Here's how the part is built. I have some questions about the finished solid (model axes, mm). Coordinates: 2 decimals unless noted, no trailing zeros. Write each loop counter-clockwise with the first axis right and the second up, starting at its lowest first coordinate (ties: lowest second). Pieces come first, ordered by that corner, then holes.
(1) Please list where these lines run through material, in increasing order: probe 1 along X at (y, z) = (-0.1, 0); probe 2 along Z at (x, y) = (0, 0.15); probe 3 along X at (y, z) = (0.3, -1.5).
(2) Imagine slicing it at B-B, the plane x = -2.5. List the corners of the cut face in (y, z) for me.
(3) Imagine slicing it at D-D, the plane x = -3.5. List the corners of the cut face in (y, z) for me, plus the area to 3 significant figures.
(4) Imagine slicing it at C-C, the plane x = 0. List the corners of the cut face in (y, z) for me.
(5) Imagine slicing it at A-A, the plane z = 1. List the corners of the cut face in (x, y) for me.
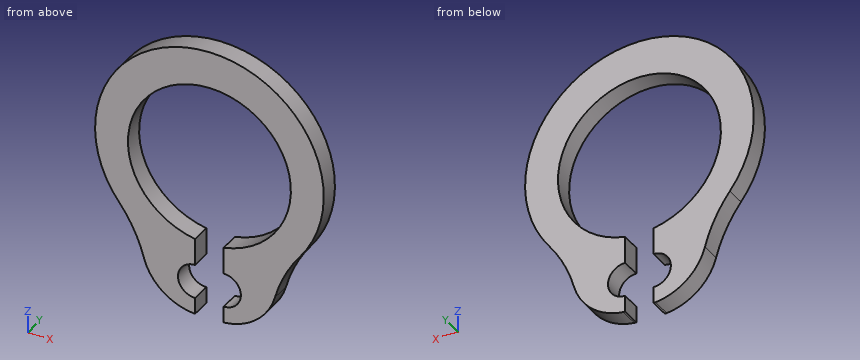
```python
from build123d import *

# Parameters (mm, degrees)
F1_DEPTH    = 0.35
F2_T1_DEPTH = 0.7
F3_R        = 2


# Not quite as in the source:
# - a fillet or chamfer that OpenCascade refuses, or shapes differently, is made with other operations: its cross-section is extruded or revolved along the edge and cut away or added


with BuildPart() as f1:
    # F0 (on Front) → F1 (new body, symmetric)
    with BuildSketch(Plane.XZ):
        with BuildLine():
            ThreePointArc((-0.5, -2.8057975693), (0, 2.85), (0.5, -2.8057975693))
            Line((0.5, -2.8057975693), (0.5, -3.75))
            ThreePointArc((0.5, -3.75), (1.1, -4.35), (0.5, -4.95))
            Line((0.5, -4.95), (0.5, -5.5274315916))
            ThreePointArc((0.5, -5.5274315916), (1.3270959738, -5.3889995617), (2.1238930496, -5.1275314054))
            Line((2.1238930496, -5.1275314054), (1.4775430927, -3.5671045734))
            ThreePointArc((1.4775430927, -3.5671045734), (0, 4.15), (-1.4775430927, -3.5671045734))
            Line((-1.4775430927, -3.5671045734), (-2.1238930496, -5.1275314054))
            ThreePointArc((-2.1238930496, -5.1275314054), (-1.3270959738, -5.3889995617), (-0.5, -5.5274315916))
            Line((-0.5, -5.5274315916), (-0.5, -4.95))
            ThreePointArc((-0.5, -4.95), (-1.1, -4.35), (-0.5, -3.75))
            Line((-0.5, -3.75), (-0.5, -2.8057975693))
        make_face()
    extrude(amount=F1_DEPTH, both=True)

    # F2: fillet of radius 5 on 2 edges, made by hand

    # F2_s2 → F2_t1 (join)
    with BuildSketch(Plane.XZ.offset(-0.35)):
        with BuildLine():
            ThreePointArc((3.163836873, -2.2974754832), (2.4254620947, -3.6322482415), (2.1238930496, -5.1275314054))
            Line((2.1238930496, -5.1275314054), (1.4775430927, -3.5671045734))
            ThreePointArc((1.4775430927, -3.5671045734), (2.4059491896, -3.0455294549), (3.163836873, -2.2974754832))
        make_face()
        with BuildLine():
            ThreePointArc((-2.1238930496, -5.1275314054), (-2.4254620947, -3.6322482415), (-3.163836873, -2.2974754832))
            ThreePointArc((-3.163836873, -2.2974754832), (-2.4059491896, -3.0455294549), (-1.4775430927, -3.5671045734))
            Line((-1.4775430927, -3.5671045734), (-2.1238930496, -5.1275314054))
        make_face()
    extrude(amount=F2_T1_DEPTH)

    # F3
    f3_edges = [f1.edges().sort_by_distance(p)[0] for p in [
        (-2.123893, 0, -5.127531),
        (2.123893, 0, -5.127531),
    ]]
    fillet(f3_edges, radius=F3_R)


solid = f1.part
```
Recorded:
1. probe 1: x = -4 to -2.85, 2.85 to 4
1. probe 2: z = 2.85 to 4.15
1. probe 3: x = -3.64 to -2.42, 2.42 to 3.64
2. outline: (-0.35, -3.44) - (0.35, -3.44) - (0.35, -1.37) - (-0.35, -1.37) - close; (-0.35, 1.37) - (0.35, 1.37) - (0.35, 3.27) - (-0.35, 3.27) - close
3. outline: (-0.35, -1.79) - (0.35, -1.79) - (0.35, 2.09) - (-0.35, 2.09) - close
3. area: 2.71 mm2
4. outline: (-0.35, 2.85) - (0.35, 2.85) - (0.35, 4.15) - (-0.35, 4.15) - close
5. outline: (-3.91, -0.35) - (-2.67, -0.35) - (-2.67, 0.35) - (-3.91, 0.35) - close; (2.67, -0.35) - (3.91, -0.35) - (3.91, 0.35) - (2.67, 0.35) - close
